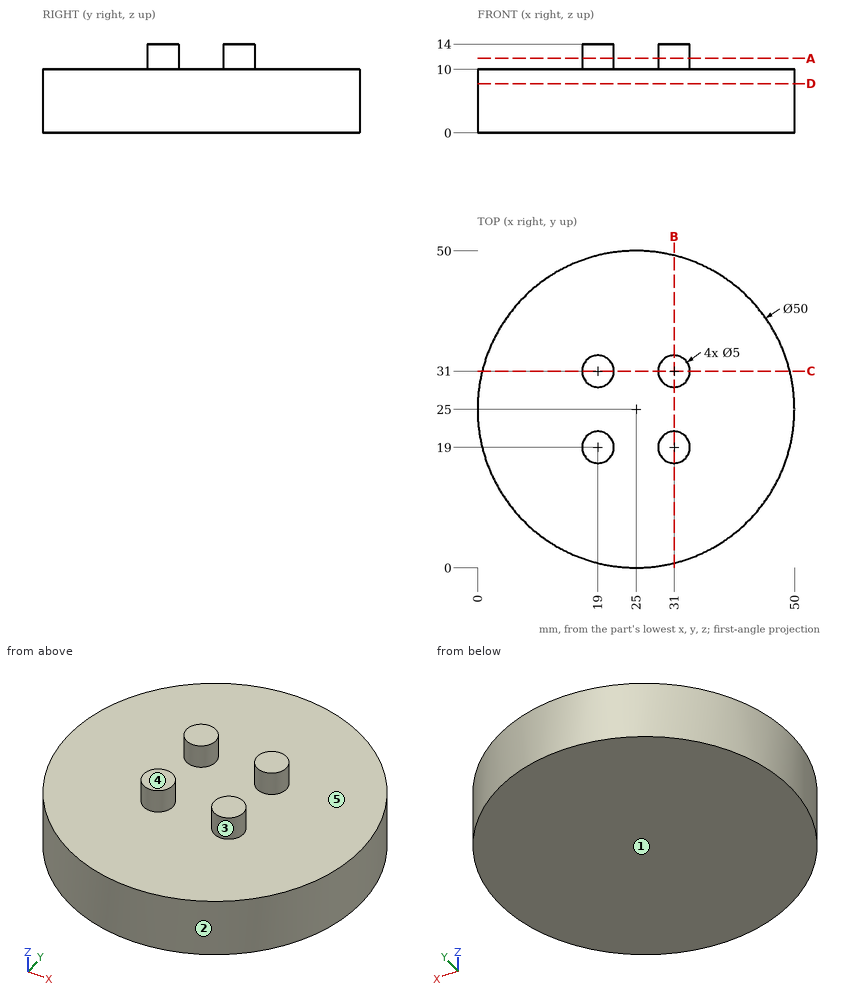
Study the drawing (mm; zero at the part's minimum x, y, z) and answer. A direction names the side the tool comes from. Give positions to 0.01 mm unless a question says otherwise; leave off trailing zeros. Loops run counter-clockwise (first coordinate to the right, second up) from the corner with the lowest first, then second, coordinate; pieces in that order, holes last. Notation, with made-up numbers: (4, 14.25) - (21, 14.25) arc R21 cw to (21, 34.25) - close; hole circle Ø7 at (2, 44.5). An arc over 180 degrees is marked (long way). Return JSON: item names as keys, results as strings. Group by question number.
1. Find section D-D (z = 7.75). Write down the section's boundary in (x, y).
2. Given pin 1 Ø5 at (x, y) = (8.5, 11) entering from +Z; pin 2 Ø1.5 at (x, z) = (42, 2.5) entering from +Y; pin 3 Ø3 at (x, z) = (35.5, 4.5) entering from -Y, each flat-ended and moving along its own axis, determine where each tip first touches the part or whether it passes through.
3. Which of the six approach directions +Z, -Z, +X, -X, +Y, -Y give full straight-line access (tool end or side, diameter ignored) to the marked faces 4 and 5?
4. Find section A-A (z = 11.75). Write down the section's boundary in (x, y).
5. Straight lines are drawn through the part: line 1 (Z direction, x = 25, y = 47.5); line 2 (Y direction, x = 2, z = 1.75); line 3 (Y direction, x = 23.5, z = 9). For each, find the intervals that lie inside material, in ascending order. Write a range as [from, to].
6. Find section B-B (x = 31). Write down the section's boundary in (y, z).
7. Determine the mould class of the marked faces 1, 2 and 3 for opening direction Y: pulls with the +Y half, pulls with the -Y half, needs draft (parallel to the pull), parting line crosses it, or undercut.
Verdict:
{
 "1": {"outline": "circle Ø50 at (25, 25)"},
 "2": {"pin 1": "stops at z = 10", "pin 2": "stops at y = 44", "pin 3": "stops at y = 1.68"},
 "3": {"face 4": "+Z, +X, -X, +Y, -Y", "face 5": "+Z"},
 "4": {"outline": "circle Ø5 at (19, 19); circle Ø5 at (19, 31); circle Ø5 at (31, 19); circle Ø5 at (31, 31)"},
 "5": {"line 1": "z = [0, 10]", "line 2": "y = [15.2, 34.8]", "line 3": "y = [0.05, 49.95]"},
 "6": {"outline": "(0.73, 0) - (49.27, 0) - (49.27, 10) - (33.5, 10) - (33.5, 14) - (28.5, 14) - (28.5, 10) - (21.5, 10) - (21.5, 14) - (16.5, 14) - (16.5, 10) - (0.73, 10) - close"},
 "7": {"face 1": "needs draft", "face 2": "parting line crosses it", "face 3": "undercut"}
}
